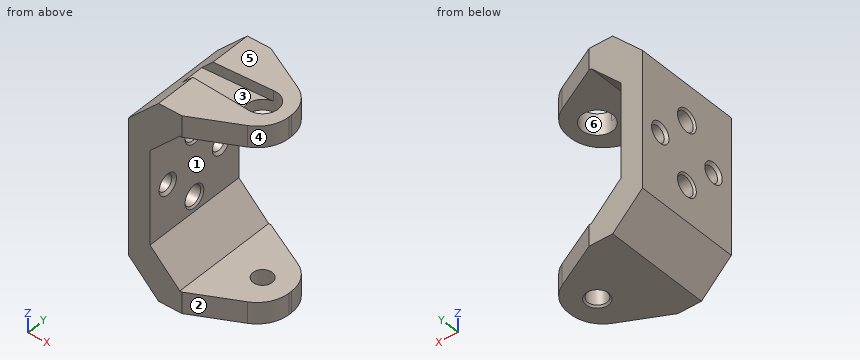
Solid Edge part; units mm, degrees
sketch "Sketch1" plane through (0, 0, 0) normal (0, -1, 0) x (1, 0, 0)
  line L0 (0, 0) -> (22.5, 0)
  line L1 (22.5, 0) -> (22.5, 5)
  line L2 (22.5, 5) -> (-5, 5)
  line L3 (-5, 5) -> (-5, -41)
  line L4 (-5, -41) -> (22.5, -41)
  line L5 (22.5, -41) -> (22.5, -36)
  line L6 (22.5, -36) -> (0, -36)
  line L7 (0, -36) -> (0, 0)
  dimension "D1" = 22.5
  dimension "D2" = 22.5
  dimension "D3" = 22.5
extrude "Protrusion1" add sketch "Sketch1" along normal mid plane 25
sketch "Sketch2" plane through (7.5, 0, 5) normal (0, 0, 1) x (0, 1, 0)
  line L0 (-12.5, 0) -> (-5, -15)
  line L1 (-5, -15) -> (5, -15)
  line L2 (5, -15) -> (12.5, 0)
  line L3 (12.5, 0) -> (12.5, -17.5)
  line L4 (12.5, -17.5) -> (-12.5, -17.5)
  line L5 (-12.5, -17.5) -> (-12.5, 0)
  dimension "D1" = 12.5
  dimension "D2" = 5
extrude "Cutout1" cut sketch "Sketch2" against normal through all
fillet "coned_rounding" radius 7.5 4 edges at (22.5, -5, 2.5) (22.5, 5, 2.5) (22.5, -5, -38.5) (22.5, 5, -38.5)
hole "Hole_2" at (16, 0, 5) direction (0, 0, -1) diameter 4.5 end through all start chamfer 0.4 start chamfer angle 45 end chamfer 0.4 end chamfer angle 45
hole "Hole_3" at (16, 0, 5) direction (0, 0, -1) diameter 7.2 end up to next
sketch "Sketch3" plane through (7.5, 0, 5) normal (0, 0, 1) x (0, 1, 0)
  line L0 (-3.6, -8.5) -> (3.6, -8.5)
  line L1 (3.6, -8.5) -> (2.4993, 11.5)
  line L2 (2.4993, 11.5) -> (-2.4993, 11.5)
  line L3 (-2.4993, 11.5) -> (-3.6, -8.5)
extrude "ExtrudedCutout_2" cut sketch "Sketch3" against normal blind 2.5
hole "Hole1" at (0, 0, -25.5) direction (-1, 0, 0) diameter 4.5 depth 30 tip angle 118 start chamfer 0.4 start chamfer angle 45 end chamfer 0.4 end chamfer angle 45
hole "Hole2" at (0, 0, -10.5) direction (-1, 0, 0) diameter 4.5 depth 30 tip angle 118 start chamfer 0.4 start chamfer angle 45 end chamfer 0.4 end chamfer angle 45
hole "Hole_8" at (0, -7.5, -18) direction (-1, 0, 0) diameter 3.7 depth 30 tip angle 118 start chamfer 0.6 start chamfer angle 45 end chamfer 0.6 end chamfer angle 45
hole "Hole3" at (0, 7.5, -18) direction (-1, 0, 0) diameter 3.7 depth 30 tip angle 118 start chamfer 0.6 start chamfer angle 45 end chamfer 0.6 end chamfer angle 45
chamfer "Chamfer_1" distance 7 angle 45 4 edges at (0, 0, -36) (-5, 0, -41) (0, 0, 0) (-5, 0, 5)
properties material "Polypropylene, general purpose"
Could you check a few things on this model? Use its own coordinates, in mm. Face numbers are marked on the shaded views. A direction names the side the tool comes from. Round coordinates to 2 decimals unless told otherwise and drop trailing zeros. Loops run counter-clockwise (first coordinate to the right, second up) from the corner with the lowest first, then second, coordinate; pieces in that order, holes last. Notation, with made-up numbers: (-7, 69) - (40, 69) arc R31 ccw to (40, 105) - close; hole circle Ø6 at (59, 86.5). An arc over 180 degrees is marked (long way). Answer as CSV lines item,"result".
1. We'd pull the mould along Y, two halves only. Please class the marked faces 3, 4, 5 and 6: +Y half, -Y half, draft (parallel to the pull), parting line (faces both ways), or undercut.
Filled in:
face 3,"undercut"
face 4,"-Y half"
face 5,"draft"
face 6,"undercut"
2. I want a section at D-D on y = 4.5. List the corners of the cut face in (x, z) for me.
Filled in:
outline,"(-5, -34) - (2, -41) - (21.26, -41) - (21.26, -36) - (7, -36) - (0, -29) - (0, -7) - (7, 0) - (21.26, 0) - (21.26, 5) - (2, 5) - (-5, -2) - close"
3. Please list where these lines run through material, in increasing order: line 1 along Y through (x, z) = (-2.95, -18); line 2 along Z through (x, y) = (9, -1); line 3 along X through (y, z) = (7, -8.5). Write a range as [from, to].
Filled in:
line 1,"y = [-12.5, -9.35], [-5.65, 5.65], [9.35, 12.5]"
line 2,"z = [-41, -36], [0, 2.5]"
line 3,"x = [-5, 0]"
4. I want a section at B-B on z = -10.5. List the corners of the cut face in (x, y) for me, then the cut area to 3 significant figures.
Filled in:
outline,"(-5, -12.5) - (0, -12.5) - (0, -2.65) - (-0.4, -2.25) - (-4.6, -2.25) - (-5, -2.65) - close; (-5, 2.65) - (-4.6, 2.25) - (-0.4, 2.25) - (0, 2.65) - (0, 12.5) - (-5, 12.5) - close"
area,"102 mm^2"
5. I want a section at A-A on z = -18. List the corners of the cut face in (x, y) for me, then the cut area to 3 significant figures.
Filled in:
outline,"(-5, -12.5) - (0, -12.5) - (0, -9.95) - (-0.6, -9.35) - (-4.4, -9.35) - (-5, -9.95) - close; (-5, -5.05) - (-4.4, -5.65) - (-0.6, -5.65) - (0, -5.05) - (0, 5.05) - (-0.6, 5.65) - (-4.4, 5.65) - (-5, 5.05) - close; (-5, 9.95) - (-4.4, 9.35) - (-0.6, 9.35) - (0, 9.95) - (0, 12.5) - (-5, 12.5) - close"
area,"86.6 mm^2"
6. On a 3-axis mill with a long thin cutter (end or side, diameter ignored), from which of +Z, -Z, +X, -X, +Y, -Y can I reach the whole of each face in a straight line? I mean the marked faces 1 and 2. Say none if no direction works.
Filled in:
face 1,"+X, +Y, -Y"
face 2,"+Z, -Z, +X, -Y"
7. I want a section at C-C on x = 6. List the corners of the cut face in (y, z) for me, then the cut area to 3 significant figures.
Filled in:
outline,"(-12.5, -41) - (12.5, -41) - (12.5, -35) - (-12.5, -35) - close; (-12.5, -1) - (12.5, -1) - (12.5, 5) - (3.05, 5) - (3.05, 2.5) - (-3.05, 2.5) - (-3.05, 5) - (-12.5, 5) - close"
area,"285 mm^2"
8. For pin 1 Ø4.5 at (y, z) = (-7.5, -18) entering from -X; pin 2 Ø4 at (x, y) = (16, 0) entering from +Z; pin 3 Ø6.5 at (y, z) = (6, -21) entering from +X; pin 4 Ø1.5 at (x, y) = (3.5, -1) entering from +Z, each with a flat end and sliding along its axis, tell me the tip position at first contact or that it passes through.
Filled in:
pin 1,"stops at x = -4.8"
pin 2,"passes through"
pin 3,"stops at x = 0"
pin 4,"stops at z = 2.5"
